Build history of the part. All positions in model axes, mm. Face numbers are marked on the shaded views. A direction names the side the tool comes from. Give positions to 0.01 mm unless a question says otherwise; leave off trailing zeros. Order: outer loops, then holes, each group sorted by start corner. A loop starts at its lowest first (then second) coordinate and runs counter-clockwise, first axis right, second up. Notation, with made-up numbers: (9, -35) -> (16, -35) arc R12 cw to (16, -27) -> close; hole circle Ø11 at (32.5, -18). An arc over 180 degrees is marked (long way). One line per item, written item: value. Start each with the question number.
(1) Saw through at B-B on z = 5. Give the cut face in (x, y).
(2) Two-plate mould, pull along X, no slides. Class the marked faces 1, 2, 3 and 4: +X half, -X half, draft (parallel to the pull), parting line (faces both ways), or undercut.
(3) Saw through at A-A on x = -34. Give the cut face in (y, z).
(4) Probe line 1 (Z direction, x = 48.05, y = 13); line 2 (Z direction, x = 28, y = -48); line 3 (X direction, y = -14, z = 33). List the from-to ranges inside material, lowest first.
(5) Which spindle directions (+Z, -Z, +X, -X, +Y, -Y) get a long thin tool onto all of the face, cutting with end or side? Do the marked faces 5 and 6. Say none if no direction does.
(6) Saw through at D-D on y = -8.5. Give the cut face in (x, z).
(7) Saw through at C-C on z = 116. Give the cut face in (x, y), plus the area to 3 significant figures.
(8) Pin check, flat tips, straight feed: pin 1 (6 mm diameter, centred on y = -31, z = 44, fed in from -X); pin 2 (6.5 mm diameter, centred on y = -37, z = 116, fed in from -X); pin 3 (5.5 mm diameter, centred on y = -28.84, z = 86.65, fed in from +X). Stop position of each tip, or through.
```python
from build123d import *

# Parameters (mm, degrees)
SKETCH1_W                      = 100
SKETCH1_H                      = 100
SKETCH1_W_2                    = 94
SKETCH1_H_2                    = 94
EXTRUDE_THIN1_DEPTH            = 130
FILLET1_R                      = 0.5
FILLET2_R                      = 3
F_8_0_8_DIAMETER_HOLE2_D       = 8
F_8_0_8_DIAMETER_HOLE3_D       = 8
F_10_0_10_DIAMETER_HOLE1_D     = 10
F_10_0_10_DIAMETER_HOLE2_D     = 10
M8_TAPPED_HOLE1_D              = 6.8
M8_TAPPED_HOLE1_DEPTH          = 3
M8_TAPPED_HOLE2_D              = 6.8
M8_TAPPED_HOLE2_DEPTH          = 3
F_21_0_21_DIAMETER_HOLE1_D     = 21
F_21_0_21_DIAMETER_HOLE1_DEPTH = 3
F_6_0_6_DIAMETER_HOLE1_D       = 6
F_6_0_6_DIAMETER_HOLE1_DEPTH   = 3
CUT_EXTRUDE1_REACH             = 173.464
SKETCH27_R                     = 2
SKETCH27_R_2                   = 3.5
CUT_EXTRUDE2_REACH             = 173.464
SKETCH31_R                     = 4


with BuildPart() as part:
    # Sketch1 → Extrude-Thin1 (new body)
    with BuildSketch(Plane.XY):
        Rectangle(SKETCH1_W, SKETCH1_H)
        Rectangle(SKETCH1_W_2, SKETCH1_H_2, mode=Mode.SUBTRACT)
    extrude(amount=EXTRUDE_THIN1_DEPTH)

    # Fillet1
    fillet1_edges = [part.edges().sort_by_distance(p)[0] for p in [
        (47, -47, 65),
        (47, 47, 65),
        (-47, 47, 65),
        (-47, -47, 65),
    ]]
    fillet(fillet1_edges, radius=FILLET1_R)

    # Fillet2
    fillet2_edges = [part.edges().sort_by_distance(p)[0] for p in [
        (50, -50, 65),
        (-50, -50, 65),
        (-50, 50, 65),
        (50, 50, 65),
    ]]
    fillet(fillet2_edges, radius=FILLET2_R)

    # Ø8.0 (8) Diameter Hole2 (through all)
    with Locations(Plane(origin=(0, 50, 0), x_dir=(1, 0, 0), z_dir=(0, 1, 0))):
        with Locations((28, -32), (28, -90)):
            Hole(F_8_0_8_DIAMETER_HOLE2_D / 2)

    # Ø8.0 (8) Diameter Hole3 (through all)
    with Locations(Plane(origin=(50, 0, 0), x_dir=(0, 0, -1), z_dir=(1, 0, 0))):
        with Locations((-14, 31), (-116, 31)):
            Hole(F_8_0_8_DIAMETER_HOLE3_D / 2)

    # Ø10.0 (10) Diameter Hole1 (through all)
    with Locations(Plane(origin=(0, 50, 0), x_dir=(1, 0, 0), z_dir=(0, 1, 0))):
        with Locations((-34, -56)):
            Hole(F_10_0_10_DIAMETER_HOLE1_D / 2)

    # Ø10.0 (10) Diameter Hole2 (through all)
    with Locations(Plane(origin=(50, 0, 0), x_dir=(0, 0, -1), z_dir=(1, 0, 0))):
        with Locations((-44, -31)):
            Hole(F_10_0_10_DIAMETER_HOLE2_D / 2)

    # M8 Tapped Hole1
    with Locations(Plane.ZY.offset(50)):
        with Locations((56, -15), (56, 35)):
            Hole(M8_TAPPED_HOLE1_D / 2, depth=M8_TAPPED_HOLE1_DEPTH)

    # M8 Tapped Hole2
    with Locations(Plane(origin=(0, -50, 0), x_dir=(-1, 0, 0), z_dir=(0, -1, 0))):
        with Locations((20, -44), (-35, -44)):
            Hole(M8_TAPPED_HOLE2_D / 2, depth=M8_TAPPED_HOLE2_DEPTH)

    # Ø21.0 (21) Diameter Hole1
    with Locations(Plane(origin=(50, 0, 0), x_dir=(0, 0, -1), z_dir=(1, 0, 0))):
        with Locations((-70, 0)):
            Hole(F_21_0_21_DIAMETER_HOLE1_D / 2, depth=F_21_0_21_DIAMETER_HOLE1_DEPTH)

    # Ø6.0 (6) Diameter Hole1
    with Locations(Plane(origin=(50, 0, 0), x_dir=(0, 0, -1), z_dir=(1, 0, 0))):
        with Locations((-41.157258279, -16.652364697), (-53.347635303, 28.842741721), (-98.842741721, 16.652364697), (-86.652364697, -28.842741721)):
            Hole(F_6_0_6_DIAMETER_HOLE1_D / 2, depth=F_6_0_6_DIAMETER_HOLE1_DEPTH)

    # Sketch27 → Cut-Extrude1 (cut, up to next)
    with BuildSketch(Plane(origin=(50, 0, 0), x_dir=(0, 0, -1), z_dir=(1, 0, 0)), mode=Mode.PRIVATE) as cut_extrude1_sk1:
        with Locations(Location((-5, 13, 0), (0, 0, 90))):
            Circle(SKETCH27_R)
    cut_extrude1_tool1 = extrude(cut_extrude1_sk1.sketch, amount=-CUT_EXTRUDE1_REACH, mode=Mode.PRIVATE) & part.part
    # Sketch27 → Cut-Extrude1 (cut, up to next)
    with BuildSketch(Plane(origin=(50, 0, 0), x_dir=(0, 0, -1), z_dir=(1, 0, 0)), mode=Mode.PRIVATE) as cut_extrude1_sk2:
        with Locations(Location((-5, 4, 0), (0, 0, 90))):
            Circle(SKETCH27_R)
    cut_extrude1_tool2 = extrude(cut_extrude1_sk2.sketch, amount=-CUT_EXTRUDE1_REACH, mode=Mode.PRIVATE) & part.part
    # Sketch27 → Cut-Extrude1 (cut, up to next)
    with BuildSketch(Plane(origin=(50, 0, 0), x_dir=(0, 0, -1), z_dir=(1, 0, 0)), mode=Mode.PRIVATE) as cut_extrude1_sk3:
        with Locations(Location((-23, 8.5, 0), (0, 0, 90))):
            Circle(SKETCH27_R_2)
    cut_extrude1_tool3 = extrude(cut_extrude1_sk3.sketch, amount=-CUT_EXTRUDE1_REACH, mode=Mode.PRIVATE) & part.part
    # Sketch27 → Cut-Extrude1 (cut, up to next)
    with BuildSketch(Plane(origin=(50, 0, 0), x_dir=(0, 0, -1), z_dir=(1, 0, 0)), mode=Mode.PRIVATE) as cut_extrude1_sk4:
        with Locations(Location((-107, 8.5, 0), (0, 0, 270))):
            Circle(SKETCH27_R_2)
    cut_extrude1_tool4 = extrude(cut_extrude1_sk4.sketch, amount=-CUT_EXTRUDE1_REACH, mode=Mode.PRIVATE) & part.part
    # Sketch27 → Cut-Extrude1 (cut, up to next)
    with BuildSketch(Plane(origin=(50, 0, 0), x_dir=(0, 0, -1), z_dir=(1, 0, 0)), mode=Mode.PRIVATE) as cut_extrude1_sk5:
        with Locations(Location((-125, 4, 0), (0, 0, 270))):
            Circle(SKETCH27_R)
    cut_extrude1_tool5 = extrude(cut_extrude1_sk5.sketch, amount=-CUT_EXTRUDE1_REACH, mode=Mode.PRIVATE) & part.part
    # Sketch27 → Cut-Extrude1 (cut, up to next)
    with BuildSketch(Plane(origin=(50, 0, 0), x_dir=(0, 0, -1), z_dir=(1, 0, 0)), mode=Mode.PRIVATE) as cut_extrude1_sk6:
        with Locations(Location((-125, 13, 0), (0, 0, 270))):
            Circle(SKETCH27_R)
    cut_extrude1_tool6 = extrude(cut_extrude1_sk6.sketch, amount=-CUT_EXTRUDE1_REACH, mode=Mode.PRIVATE) & part.part
    add(cut_extrude1_tool1.solids().sort_by_distance((50, 13, 5))[0], mode=Mode.SUBTRACT)
    add(cut_extrude1_tool2.solids().sort_by_distance((50, 4, 5))[0], mode=Mode.SUBTRACT)
    add(cut_extrude1_tool3.solids().sort_by_distance((50, 8.5, 23))[0], mode=Mode.SUBTRACT)
    add(cut_extrude1_tool4.solids().sort_by_distance((50, 8.5, 107))[0], mode=Mode.SUBTRACT)
    add(cut_extrude1_tool5.solids().sort_by_distance((50, 4, 125))[0], mode=Mode.SUBTRACT)
    add(cut_extrude1_tool6.solids().sort_by_distance((50, 13, 125))[0], mode=Mode.SUBTRACT)

    # Sketch31 → Cut-Extrude2 (cut, up to next)
    with BuildSketch(Plane.ZY.offset(50), mode=Mode.PRIVATE) as cut_extrude2_sk1:
        with Locations(Location((14, -37, 0), (0, 0, 270))):
            Circle(SKETCH31_R)
    cut_extrude2_tool1 = extrude(cut_extrude2_sk1.sketch, amount=-CUT_EXTRUDE2_REACH, mode=Mode.PRIVATE) & part.part
    # Sketch31 → Cut-Extrude2 (cut, up to next)
    with BuildSketch(Plane.ZY.offset(50), mode=Mode.PRIVATE) as cut_extrude2_sk2:
        with Locations(Location((116, -37, 0), (0, 0, 270))):
            Circle(SKETCH31_R)
    cut_extrude2_tool2 = extrude(cut_extrude2_sk2.sketch, amount=-CUT_EXTRUDE2_REACH, mode=Mode.PRIVATE) & part.part
    add(cut_extrude2_tool1.solids().sort_by_distance((-50, -37, 14))[0], mode=Mode.SUBTRACT)
    add(cut_extrude2_tool2.solids().sort_by_distance((-50, -37, 116))[0], mode=Mode.SUBTRACT)


solid = part.part
```
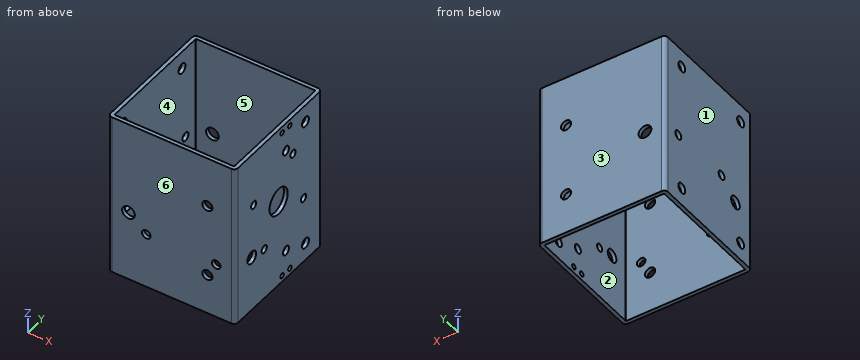
Results below:
1. outline: (-50, -47) arc R3 ccw to (-47, -50) -> (47, -50) arc R3 ccw to (50, -47) -> (50, 2) -> (47, 2) -> (47, -46.5) arc R0.5 cw to (46.5, -47) -> (-46.5, -47) arc R0.5 cw to (-47, -46.5) -> (-47, 46.5) arc R0.5 cw to (-46.5, 47) -> (46.5, 47) arc R0.5 cw to (47, 46.5) -> (47, 15) -> (50, 15) -> (50, 47) arc R3 ccw to (47, 50) -> (-47, 50) arc R3 ccw to (-50, 47) -> close; (47, 6) -> (50, 6) -> (50, 11) -> (47, 11) -> close
2. face 1: -X half
2. face 2: undercut
2. face 3: draft
2. face 4: undercut
3. outline: (-50, 0) -> (-47, 0) -> (-47, 51) -> (-50, 51) -> close; (-50, 61) -> (-47, 61) -> (-47, 130) -> (-50, 130) -> close; (47, 0) -> (50, 0) -> (50, 51) -> (47, 51) -> close; (47, 61) -> (50, 61) -> (50, 130) -> (47, 130) -> close
4. line 1: z = 0 to 3, 7 to 123, 127 to 130
4. line 2: z = 0 to 28, 36 to 86, 94 to 130
4. line 3: x = -50 to -47, 47 to 50
5. face 5: +Z, -Z
5. face 6: +Z, -Z, +X, -X, -Y
6. outline: (-50, 0) -> (-47, 0) -> (-47, 130) -> (-50, 130) -> close; (47, 0) -> (50, 0) -> (50, 63.84) -> (47, 63.84) -> close; (47, 76.16) -> (50, 76.16) -> (50, 130) -> (47, 130) -> close
7. outline: (-50, -47) arc R3 ccw to (-47, -50) -> (47, -50) arc R3 ccw to (50, -47) -> (50, 27) -> (47, 27) -> (47, -46.5) arc R0.5 cw to (46.5, -47) -> (-46.5, -47) arc R0.5 cw to (-47, -46.5) -> (-47, -41) -> (-50, -41) -> close; (-50, -33) -> (-47, -33) -> (-47, 27) -> (-50, 27) -> close; (-50, 35) -> (-47, 35) -> (-47, 46.5) arc R0.5 cw to (-46.5, 47) -> (46.5, 47) arc R0.5 cw to (47, 46.5) -> (47, 35) -> (50, 35) -> (50, 47) arc R3 ccw to (47, 50) -> (-47, 50) arc R3 ccw to (-50, 47) -> close
7. area: 1,080 mm²
8. pin 1: passes through
8. pin 2: stops at x = 47
8. pin 3: stops at x = -47
